The listing builds one solid part. Answer for the finished solid, in the listing's coordinates (mm). A direction names the side the tool comes from. Give positions to 0.01 mm unless a question says otherwise; leave off trailing zeros. Write each loop counter-clockwise with the first axis right and the second up, starting at its lowest first coordinate (ties: lowest second). Pieces come first, ordered by that corner, then holes. Notation, with made-up numbers: (-5.75, 9) - (16.25, 9) arc R17 ccw to (16.25, 27) - close; hole circle Ø3 at (-8.5, 61.5). An arc over 180 degrees is marked (long way). One line per question, with ' | ' between items. Start each with the question number.
1. Given P1, Ø2.5, axis at x = -12.5, y = -1.5, coming from the -Z side (3 decimals); P2, Ø2.5, axis at y = 1, z = -14.5, coming from the -X side (3 decimals); P3, Ø1.6, axis at x = 72.5, y = 2, coming from the +Z side (3 decimals); P4, Ø0.8, axis at x = 74.93, z = 0, coming from the -Y side, each flat-ended and moving along its own axis, determine where each tip first touches the part or whether it passes through.
2. Find the intervals of material crossed by L1, parallel to Z at x = 26.5, y = 2 (3 decimals); L2, parallel to X at y = 0.5, z = 13; L3, parallel to Y at x = 23, z = 9.5, in increasing order. Write a range as from..to.
3. A cutting plane is placed at C-C (x = -13.5). Determine the outline of the cut face in (y, z) (3 decimals), then the cut area to 3 significant figures.
4. The mould has two halves that part along X. Classify faces 4 (the face through (73.66, 1, 10)), 5 (the face through (76.2, 0, -15)), 6 (the face through (-63.322, 0.053, -16.053)), 7 (the face through (-61.537, 1.306, -14.246)): +X half, -X half, draft (parallel to the pull), parting line (faces both ways), or undercut.
5. A cutting plane is placed at B-B (z = 13.5). Determine the outline of the cut face in (x, y).
6. For faces 1 (the face through (-76.2, 0, 12)), 2 (the face through (69.149, 1.234, -42.062)), 3 (the face through (6, 0, -28.575)), determine the directions among +Z, -Z, +X, -X, +Y, -Y from which every point of the face is accessible in a straight line to the end or side of a thin tool.
7. A cutting plane is placed at A-A (y = 2.25). Determine the outline of the cut face in (x, z) (3 decimals), then the cut area to 3 significant figures.
```python
from build123d import *

# Parameters (mm, degrees)
F0_W     = 152.4
F0_H     = 57.15
F0_R     = 0.635
F1_DEPTH = 3.81
F2_SIZE  = 25.4
F3_W     = 12.7
F3_H     = 19.05
F4_DEPTH = 7.62
F5_SIZE  = 7.62
F6_SIZE  = 10.16
F7_T     = -2.54


with BuildPart() as f1:
    # F0 (on Front) → F1 (new body, symmetric)
    with BuildSketch(Plane.XZ):
        Rectangle(F0_W, F0_H)
        with Locations((74.9251618981, 0)):
            Circle(F0_R, mode=Mode.SUBTRACT)
    extrude(amount=F1_DEPTH, both=True)

    # F2
    f2_edges = [f1.edges().sort_by_distance(p)[0] for p in [
        (-76.2, 0, -28.575),
    ]]
    chamfer(f2_edges, length=F2_SIZE)

    # F3 (on face) → F4 (join)
    with BuildSketch(Plane.XZ.offset(3.81)):
        with Locations((69.85, -38.1)):
            Rectangle(F3_W, F3_H)
    extrude(amount=-F4_DEPTH)

    # F5
    f5_edges = [f1.edges().sort_by_distance(p)[0] for p in [
        (63.5, 0, -47.625),
    ]]
    chamfer(f5_edges, length=F5_SIZE)

    # F6
    f6_edges = [f1.edges().sort_by_distance(p)[0] for p in [
        (76.2, 0, 28.575),
    ]]
    chamfer(f6_edges, length=F6_SIZE)

    # F7
    f7_openings = [f1.faces().sort_by_distance(p)[0] for p in [
        (3.858416, 3.81, -0.318506),
    ]]
    offset(amount=F7_T, openings=f7_openings, kind=Kind.INTERSECTION)


solid = f1.part
```
Determined:
1) P1: z = -28.575 | P2: x = -66.125 | P3: z = 22.915 | P4: through
2) L1: -28.575..-26.035, 26.035..28.575 | L2: -76.2..-73.66, 73.66..76.2 | L3: -3.81..-1.27
3) outline: (-3.81, -28.575) - (3.81, -28.575) - (3.81, -26.035) - (-1.27, -26.035) - (-1.27, 26.035) - (3.81, 26.035) - (3.81, 28.575) - (-3.81, 28.575) - close | area: 171 mm2
4) face 4: undercut | face 5: +X half | face 6: -X half | face 7: undercut
5) outline: (-76.2, -3.81) - (76.2, -3.81) - (76.2, 3.81) - (73.66, 3.81) - (73.66, -1.27) - (-73.66, -1.27) - (-73.66, 3.81) - (-76.2, 3.81) - close
6) face 1: +Z, -Z, -X, +Y, -Y | face 2: +Y | face 3: -Z, -X, +Y, -Y
7) outline: (-76.2, -3.175) - (-50.8, -28.575) - (63.5, -28.575) - (63.5, -40.005) - (71.12, -47.625) - (76.2, -47.625) - (76.2, 18.415) - (66.04, 28.575) - (-76.2, 28.575) - close; hole (-73.66, -2.123) - (-49.748, -26.035) - (66.04, -26.035) - (66.04, -38.953) - (72.172, -45.085) - (73.66, -45.085) - (73.66, -2.912) arc R3.175 cw to (73.66, 2.912) - (73.66, 17.363) - (64.988, 26.035) - (-73.66, 26.035) - close; hole circle Ø1.27 at (74.925, 0) | area: 1,080 mm2
